from build123d import *

# Parameters (mm, degrees)
SKETCH1_W           = 71
SKETCH1_H           = 50
SKETCH1_R           = 2.125
BOSS_EXTRUDE1_DEPTH = 3
SKETCH2_W           = 77
SKETCH2_H           = 56
SKETCH2_W_2         = 71
SKETCH2_H_2         = 50
BOSS_EXTRUDE2_DEPTH = 30
SKETCH3_W           = 71
SKETCH3_H           = 30
CUT_EXTRUDE1_DEPTH  = 75.284924446
CUT_EXTRUDE2_DEPTH  = 88.252507127
FILLET1_R           = 3


with BuildPart() as part:
    # Sketch1 → Boss-Extrude1 (new body)
    with BuildSketch(Plane(origin=(0, 0, 0), x_dir=(1, 0, 0), z_dir=(0, 1, 0))):
        Rectangle(SKETCH1_W, SKETCH1_H)
        with Locations(Location((-31.5, 21, 0), (0, 0, 270))):
            Circle(SKETCH1_R, mode=Mode.SUBTRACT)
        with Locations(Location((31.5, 21, 0), (0, 0, 270))):
            Circle(SKETCH1_R, mode=Mode.SUBTRACT)
        with Locations(Location((31.5, -21, 0), (0, 0, 270))):
            Circle(SKETCH1_R, mode=Mode.SUBTRACT)
        with Locations(Location((-31.5, -21, 0), (0, 0, 270))):
            Circle(SKETCH1_R, mode=Mode.SUBTRACT)
    extrude(amount=BOSS_EXTRUDE1_DEPTH)

    # Sketch2 → Boss-Extrude2 (add)
    with BuildSketch(Plane(origin=(0, 0, 0), x_dir=(1, 0, 0), z_dir=(0, 1, 0))):
        Rectangle(SKETCH2_W, SKETCH2_H)
        Rectangle(SKETCH2_W_2, SKETCH2_H_2, mode=Mode.SUBTRACT)
    extrude(amount=BOSS_EXTRUDE2_DEPTH)

    # Sketch3 → Cut-Extrude1 (cut, through all)
    with BuildSketch(Plane(origin=(0, 0, -28), x_dir=(-1, 0, 0), z_dir=(0, 0, -1))):
        with Locations((0, 24)):
            Rectangle(SKETCH3_W, SKETCH3_H)
    extrude(amount=-CUT_EXTRUDE1_DEPTH, mode=Mode.SUBTRACT)

    # Sketch4 → Cut-Extrude2 (cut, through all)
    with BuildSketch(Plane.ZY.offset(38.5)):
        with BuildLine():
            Line((-18, 24), (-23, 24))
            ThreePointArc((-23, 24), (-25, 26), (-23, 28))
            Line((-23, 28), (-18, 28))
            ThreePointArc((-18, 28), (-16, 26), (-18, 24))
        make_face()
        with BuildLine():
            Line((2, 28), (-3, 28))
            ThreePointArc((-3, 28), (-5, 26), (-3, 24))
            Line((-3, 24), (2, 24))
            ThreePointArc((2, 24), (4, 26), (2, 28))
        make_face()
        with BuildLine():
            Line((22, 28), (17, 28))
            ThreePointArc((17, 28), (15, 26), (17, 24))
            Line((17, 24), (22, 24))
            ThreePointArc((22, 24), (24, 26), (22, 28))
        make_face()
    extrude(amount=-CUT_EXTRUDE2_DEPTH, mode=Mode.SUBTRACT)

    # Fillet1
    fillet1_edges = [part.edges().sort_by_distance(p)[0] for p in [
        (37, 30, -28),
        (-37, 30, 28),
        (37, 30, 28),
        (-37, 30, -28),
        (35.5, 9, -26.5),
        (-35.5, 9, -26.5),
        (35.5, 9, 26.5),
        (-35.5, 9, 26.5),
    ]]
    fillet(fillet1_edges, radius=FILLET1_R)


solid = part.part
Model file for the job. Use its own axes, mm. A direction names the side the tool comes from. Give positions to 0.01 mm unless a question says otherwise; leave off trailing zeros. Order: outer loops, then holes, each group sorted by start corner. A loop starts at its lowest first (then second) coordinate and runs counter-clockwise, first axis right, second up. Notation, with made-up numbers: (67, -13.75) - (99, -13.75) arc R17 cw to (99, 0.25) - close; hole circle Ø11 at (-36.75, -12). An arc over 180 degrees is marked (long way). Return JSON: item names as keys, results as strings.
1) Cut at D-D, the plane y = 26. Count the separate pieces of the cut face and the enclosed holes in it, plus the area to 3 significant figures.
Geometry says:
{"separate pieces": "8", "enclosed holes": "0", "area": "174 mm²"}
2) 3-axis set-ups, long thin cutter, end or side, ignore diameter. For faces 1 (the cylindrical face through (-32.79, 1.48, -22.69)), 2 (the flat face through (-35.5, 16, 0)), 3 (the cylindrical face through (-34.64, 9.9, -26.48)), 4 (the flat face through (38.5, 15, 0)), 5 (the cylindrical face through (37, 26, -25)): which of +Z, -Z, +X, -X, +Y, -Y reach the whole face in a straight line?
Geometry says:
{"face 1": "+Y, -Y", "face 2": "+Y", "face 3": "+Z, -Z, +Y", "face 4": "+Z, -Z, +X, +Y, -Y", "face 5": "+X, -X"}
3) Flat gauge pins, fed straight in: P1, Ø4, axis at x = 31.5, z = 21, coming from the +Y side; P2, Ø1.5, axis at x = 0, z = 26.5, coming from the +Y side. Where does each tip first touch, or does it go through?
Geometry says:
{"P1": "through", "P2": "y = 9"}
4) Probe line 1 (X direction, y = 0.6, z = -21) (3 decimals); line 2 (Z direction, x = -10, y = 6); line 3 (X direction, y = 20.75, z = 3). List the from-to ranges inside material, lowest first. Write a range as from..to.
Geometry says:
{"line 1": "-38.5..-33.625, -29.375..29.375, 33.625..38.5", "line 2": "-28..-25, 25..28", "line 3": "-38.5..-35.5, 35.5..38.5"}
5) Cut at A-A, the plane z = 21. Give the cut face in (x, y) (3 decimals).
Geometry says:
{"outline": "(-38.5, 0) - (-33.625, 0) - (-33.625, 3) - (-35.5, 3) - (-35.5, 24) - (-38.5, 24) - close; (-38.5, 28) - (-35.5, 28) - (-35.5, 30) - (-38.5, 30) - close; (-29.375, 0) - (29.375, 0) - (29.375, 3) - (-29.375, 3) - close; (33.625, 0) - (38.5, 0) - (38.5, 24) - (35.5, 24) - (35.5, 3) - (33.625, 3) - close; (35.5, 28) - (38.5, 28) - (38.5, 30) - (35.5, 30) - close"}
6) Cut at B-B, the plane x = 31.5. Give the cut face in (y, z) (3 decimals).
Geometry says:
{"outline": "(0, -28) - (9, -28) - (9, -25) - (3, -25) - (3, -23.125) - (0, -23.125) - close; (0, -18.875) - (3, -18.875) - (3, 18.875) - (0, 18.875) - close; (0, 23.125) - (3, 23.125) - (3, 25) - (9, 25) - (9, 28) - (0, 28) - close"}
7) Pull direction Y, two halves, no side cores. Call faces 6 (the cylindrical face through (30.21, 1.48, 19.31)), 7 (the cylindrical face through (37.02, 29.1, 27.14)), 8 (the flat face through (37, 28, 20)): pulls with the +Y half, pulls with the -Y half, needs draft (parallel to the pull), parting line crosses it, or undercut.
Geometry says:
{"face 6": "needs draft", "face 7": "pulls with the +Y half", "face 8": "undercut"}
8) Cut at C-C, the plane y = 17. Give the cut face in (x, z).
Geometry says:
{"outline": "(-38.5, -28) - (-35.5, -28) - (-35.5, 28) - (-38.5, 28) - close; (35.5, -28) - (38.5, -28) - (38.5, 28) - (35.5, 28) - close"}
